```python
from build123d import *

# Parameters (mm, degrees)
F0_W     = 45
F0_H     = 45
F1_DEPTH = 475
F2_W     = 15
F2_H     = 80
F2_W_2   = 30
F2_H_2   = 30
F3_DEPTH = 15


with BuildPart() as f1:
    # F0 (on Top) → F1 (new body, symmetric)
    with BuildSketch(Plane.XY):
        Rectangle(F0_W, F0_H)
    extrude(amount=F1_DEPTH, both=True)

    # F2 (on face) → F3 (cut)
    with BuildSketch(Plane.YZ.offset(22.5)):
        with Locations((0, 405)):
            Rectangle(F2_W, F2_H)
        with Locations((0, 40)):
            Rectangle(F2_W_2, F2_H_2)
    extrude(amount=-F3_DEPTH, mode=Mode.SUBTRACT)


solid = f1.part
```
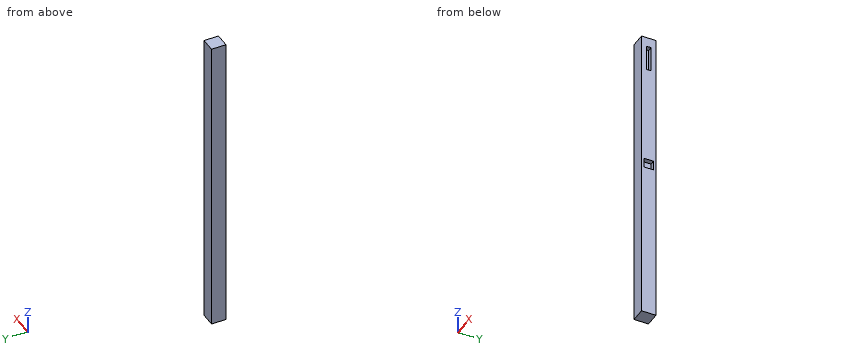
The model under review builds one solid part; all positions refer to its coordinate system, in mm. Round coordinates to 2 decimals unless told otherwise and drop trailing zeros. Order: outer loops, then holes, each group sorted by start corner. A loop starts at its lowest first (then second) coordinate and runs counter-clockwise, first axis right, second up. Notation, with made-up numbers: (37.5, 76) -> (55.5, 76) arc R22 cw to (55.5, 88) -> close; hole circle Ø8 at (-28, 82). An arc over 180 degrees is marked (long way). One line per item, written item: value. Start each with the question number.
Q1. Take a section at B-B (z = 410). Write out the cut boundary in (x, y), and give its area (3 significant figures).
Q2. Wall thickness on line 1 (Z direction, x = 17.5, y = -6); line 2 (Z direction, x = 19, y = 8): over which ranges is each line inside the solid? List them lowest first.
Q3. Take a section at A-A (z = 45). Write out the cut boundary in (x, y).
Q4. Clearance check with a flat-ended pin moving along its axis: pin 1 Ø15 at (y, z) = (-4, 38.5) entering from +X. State where the tip first meets the part, or that it passes through.
Reported:
1. outline: (-22.5, -22.5) -> (22.5, -22.5) -> (22.5, -7.5) -> (7.5, -7.5) -> (7.5, 7.5) -> (22.5, 7.5) -> (22.5, 22.5) -> (-22.5, 22.5) -> close
1. area: 1,800 mm2
2. line 1: z = -475 to 25, 55 to 365, 445 to 475
2. line 2: z = -475 to 25, 55 to 475
3. outline: (-22.5, -22.5) -> (22.5, -22.5) -> (22.5, -15) -> (7.5, -15) -> (7.5, 15) -> (22.5, 15) -> (22.5, 22.5) -> (-22.5, 22.5) -> close
4. pin 1: stops at x = 7.5
